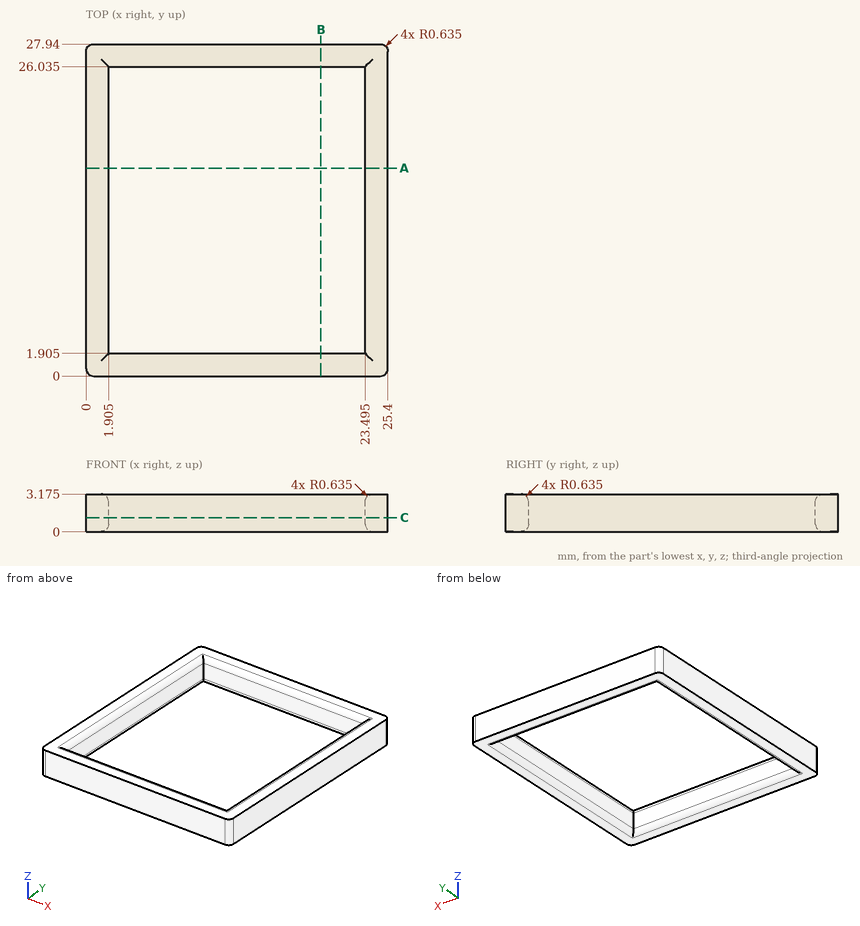
Could you check a few things on this drawing? It's one solid part, dimensions in mm from its lowest x, y, z. Coordinates: 2 decimals unless noted, no trailing zeros. Order: outer loops, then holes, each group sorted by start corner. A loop starts at its lowest first (then second) coordinate and runs counter-clockwise, first axis right, second up. Notation, with made-up numbers: (-1.75, -38) -> (15.25, -38) arc R23 cw to (15.25, -9) -> close; hole circle Ø8 at (-4.5, 75). An arc over 180 degrees is marked (long way). Answer in a Markdown table with one row per item.
(1) Will this pin go through, and if not, where does the flat tip stop? pin 1 Ø6 at (x, y) = (20, 10) entering from -Z.
Answer key:
| item | result |
|---|---|
| pin 1 | through |
(2) I want a section at B-B on x = 19.75. List the corners of the cut face in (y, z) for me (3 decimals), then the cut area to 3 significant figures.
Answer key:
| item | result |
|---|---|
| outline | (0, 0) -> (1.27, 0) arc R0.635 ccw to (1.905, 0.635) -> (1.905, 2.54) arc R0.635 ccw to (1.27, 3.175) -> (0, 3.175) -> close; (26.035, 0.635) arc R0.635 ccw to (26.67, 0) -> (27.94, 0) -> (27.94, 3.175) -> (26.67, 3.175) arc R0.635 ccw to (26.035, 2.54) -> close |
| area | 11.8 mm^2 |
(3) I want a section at A-A on y = 17.5. List the corners of the cut face in (x, z) for me (3 decimals).
Answer key:
| item | result |
|---|---|
| outline | (0, 0) -> (1.27, 0) arc R0.635 ccw to (1.905, 0.635) -> (1.905, 2.54) arc R0.635 ccw to (1.27, 3.175) -> (0, 3.175) -> close; (23.495, 0.635) arc R0.635 ccw to (24.13, 0) -> (25.4, 0) -> (25.4, 3.175) -> (24.13, 3.175) arc R0.635 ccw to (23.495, 2.54) -> close |
(4) I want a section at C-C on z = 1.2. List the corners of the cut face in (x, y) for me (3 decimals), then the cut area to 3 significant figures.
Answer key:
| item | result |
|---|---|
| outline | (0, 0.635) arc R0.635 ccw to (0.635, 0) -> (24.765, 0) arc R0.635 ccw to (25.4, 0.635) -> (25.4, 27.305) arc R0.635 ccw to (24.765, 27.94) -> (0.635, 27.94) arc R0.635 ccw to (0, 27.305) -> close; hole (1.905, 1.905) -> (23.495, 1.905) -> (23.495, 26.035) -> (1.905, 26.035) -> close |
| area | 188 mm^2 |
(5) Please list where these lines run through material, in increasing order: probe 1 along Y at (x, z) = (2.25, 1.7) (3 decimals); probe 2 along X at (y, z) = (5, 1.95) (3 decimals); probe 3 along X at (y, z) = (16.5, 0.25).
Answer key:
| item | result |
|---|---|
| probe 1 | 0 to 1.905, 26.035 to 27.94 |
| probe 2 | 0 to 1.905, 23.495 to 25.4 |
| probe 3 | 0 to 1.77, 23.63 to 25.4 |
